from build123d import *

# Parameters (mm, degrees)
F0_R      = 3.1
F0_R_2    = 2.4
F1_DEPTH  = 87.8
F2_DEPTH  = 1
F3_DEPTH  = 8
F4_R      = 2.4
F5_DEPTH  = 25
F4_R_2    = 3.1
F6_DEPTH  = 1
F7_R      = 3.1
F7_R_2    = 2.4
F8_DEPTH  = 1
F9_R      = 2.4
F10_DEPTH = 8
F9_R_2    = 3.1
F11_DEPTH = 1
F12_DEPTH = 7
F13_R     = 2.4
F14_DEPTH = 7.9
F13_R_2   = 3.1
F15_DEPTH = 1


# Not quite as in the source:
# - a pattern or mirror of a feature is missing from the dataset's text; its kind, count and spacing are read off the source's solid


with BuildPart() as f1:
    # F0 (on Front) → F1 (new body)
    with BuildSketch(Plane.XZ):
        Polygon((4, 7.8), (0, 7.8), (-4, 7.8), (-11.9, 7.8), (-11.9, 0), (0, 0), (11.9, 0), (11.9, 7.8), align=None)
        with Locations((-7.975, 3.9)):
            Circle(F0_R, mode=Mode.SUBTRACT)
        with Locations((0, 3.9)):
            Circle(F0_R, mode=Mode.SUBTRACT)
        with Locations((7.975, 3.9)):
            Circle(F0_R, mode=Mode.SUBTRACT)
        with Locations((7.975, 3.9)):
            Circle(F0_R)
        with Locations((7.975, 3.9)):
            Circle(F0_R_2, mode=Mode.SUBTRACT)
        with Locations((0, 3.9)):
            Circle(F0_R)
        with Locations((0, 3.9)):
            Circle(F0_R_2, mode=Mode.SUBTRACT)
        with Locations((-7.975, 3.9)):
            Circle(F0_R)
        with Locations((-7.975, 3.9)):
            Circle(F0_R_2, mode=Mode.SUBTRACT)
        with Locations((-7.975, 3.9)):
            Circle(F0_R_2)
        with Locations((0, 3.9)):
            Circle(F0_R_2)
        with Locations((7.975, 3.9)):
            Circle(F0_R_2)
    extrude(amount=F1_DEPTH)

    # F0 (on Front) → F2 (cut)
    with BuildSketch(Plane.XZ):
        with Locations((7.975, 3.9)):
            Circle(F0_R)
        with Locations((7.975, 3.9)):
            Circle(F0_R_2, mode=Mode.SUBTRACT)
        with Locations((0, 3.9)):
            Circle(F0_R)
        with Locations((0, 3.9)):
            Circle(F0_R_2, mode=Mode.SUBTRACT)
        with Locations((-7.975, 3.9)):
            Circle(F0_R)
        with Locations((-7.975, 3.9)):
            Circle(F0_R_2, mode=Mode.SUBTRACT)
    extrude(amount=F2_DEPTH, mode=Mode.SUBTRACT)

    # F0 (on Front) → F3 (cut)
    with BuildSketch(Plane.XZ):
        with Locations((-7.975, 3.9)):
            Circle(F0_R_2)
        with Locations((0, 3.9)):
            Circle(F0_R_2)
        with Locations((7.975, 3.9)):
            Circle(F0_R_2)
    extrude(amount=F3_DEPTH, mode=Mode.SUBTRACT)

    # F4 (on face) → F5 (cut)
    with BuildSketch(Plane.XY.offset(7.8)):
        with Locations((-7.9, -11.9)):
            Circle(F4_R)
        with Locations((-7.9, -75.9)):
            Circle(F4_R)
        with Locations((7.9, -75.9)):
            Circle(F4_R)
        with Locations((7.9, -11.9)):
            Circle(F4_R)
    extrude(amount=-F5_DEPTH, mode=Mode.SUBTRACT)

    # F4 (on face) → F6 (cut)
    with BuildSketch(Plane.XY.offset(7.8)):
        with Locations((-7.9, -11.9)):
            Circle(F4_R_2)
        with Locations((-7.9, -11.9)):
            Circle(F4_R, mode=Mode.SUBTRACT)
        with Locations((7.9, -11.9)):
            Circle(F4_R_2)
        with Locations((7.9, -11.9)):
            Circle(F4_R, mode=Mode.SUBTRACT)
        with Locations((-7.9, -75.9)):
            Circle(F4_R_2)
        with Locations((-7.9, -75.9)):
            Circle(F4_R, mode=Mode.SUBTRACT)
        with Locations((7.9, -75.9)):
            Circle(F4_R_2)
        with Locations((7.9, -75.9)):
            Circle(F4_R, mode=Mode.SUBTRACT)
    extrude(amount=-F6_DEPTH, mode=Mode.SUBTRACT)

    # F7 (on face) → F8 (cut)
    with BuildSketch(Plane(origin=(0, 0, 0), x_dir=(1, 0, 0), z_dir=(0, 0, -1))):
        with Locations((7.9, 75.9)):
            Circle(F7_R)
        with Locations((7.9, 75.9)):
            Circle(F7_R_2, mode=Mode.SUBTRACT)
        with Locations((-7.9, 75.9)):
            Circle(F7_R)
        with Locations((-7.9, 75.9)):
            Circle(F7_R_2, mode=Mode.SUBTRACT)
        with Locations((-7.9, 11.9)):
            Circle(F7_R)
        with Locations((-7.9, 11.9)):
            Circle(F7_R_2, mode=Mode.SUBTRACT)
        with Locations((7.9, 11.9)):
            Circle(F7_R)
        with Locations((7.9, 11.9)):
            Circle(F7_R_2, mode=Mode.SUBTRACT)
    extrude(amount=-F8_DEPTH, mode=Mode.SUBTRACT)

    # F9 (on face) → F10 (cut)
    with BuildSketch(Plane.YZ.offset(11.9)):
        with Locations((-67.9, 3.9)):
            Circle(F9_R)
        with Locations((-59.9, 3.9)):
            Circle(F9_R)
        with Locations((-51.9, 3.9)):
            Circle(F9_R)
        with Locations((-43.9, 3.9)):
            Circle(F9_R)
        with Locations((-35.9, 3.9)):
            Circle(F9_R)
        with Locations((-27.9, 3.9)):
            Circle(F9_R)
        with Locations((-19.9, 3.9)):
            Circle(F9_R)
    f10 = extrude(amount=-F10_DEPTH, mode=Mode.SUBTRACT)

    # F10_copies: F10 across plane
    add(f10.mirror(Plane(origin=(0, 0, 0), x_dir=(0, 0, -1), z_dir=(-1, 0, 0))), mode=Mode.SUBTRACT)

    # F9 (on face) → F11 (cut)
    with BuildSketch(Plane.YZ.offset(11.9)):
        with Locations((-67.9, 3.9)):
            Circle(F9_R_2)
        with Locations((-67.9, 3.9)):
            Circle(F9_R, mode=Mode.SUBTRACT)
        with Locations((-59.9, 3.9)):
            Circle(F9_R_2)
        with Locations((-59.9, 3.9)):
            Circle(F9_R, mode=Mode.SUBTRACT)
        with Locations((-51.9, 3.9)):
            Circle(F9_R_2)
        with Locations((-51.9, 3.9)):
            Circle(F9_R, mode=Mode.SUBTRACT)
        with Locations((-43.9, 3.9)):
            Circle(F9_R_2)
        with Locations((-43.9, 3.9)):
            Circle(F9_R, mode=Mode.SUBTRACT)
        with Locations((-35.9, 3.9)):
            Circle(F9_R_2)
        with Locations((-35.9, 3.9)):
            Circle(F9_R, mode=Mode.SUBTRACT)
        with Locations((-27.9, 3.9)):
            Circle(F9_R_2)
        with Locations((-27.9, 3.9)):
            Circle(F9_R, mode=Mode.SUBTRACT)
        with Locations((-19.9, 3.9)):
            Circle(F9_R_2)
        with Locations((-19.9, 3.9)):
            Circle(F9_R, mode=Mode.SUBTRACT)
    f11 = extrude(amount=-F11_DEPTH, mode=Mode.SUBTRACT)

    # F11_copies: F11 across plane
    add(f11.mirror(Plane(origin=(0, 0, 0), x_dir=(0, 0, -1), z_dir=(-1, 0, 0))), mode=Mode.SUBTRACT)

    # F4 (on face) → F12 (cut)
    with BuildSketch(Plane.XY.offset(7.8)):
        Polygon((-11.1, -6.9), (-11.1, -7.9), (-3.9, -7.9), (-3.9, -15.9), (-4.9, -15.9), (-4.9, -71.9), (-3.9, -71.9), (-3.9, -79.9), (-11.1, -79.9), (-11.1, -80.9), (11.1, -80.9), (11.1, -79.9), (3.9, -79.9), (3.9, -71.9), (4.9, -71.9), (4.9, -15.9), (3.9, -15.9), (3.9, -7.9), (11.1, -7.9), (11.1, -6.9), align=None)
    extrude(amount=-F12_DEPTH, mode=Mode.SUBTRACT)

    # F13 (on face) → F14 (cut)
    with BuildSketch(Plane.XZ.offset(87.8)):
        with Locations((-8, 3.9)):
            Circle(F13_R)
        with Locations((0, 3.9)):
            Circle(F13_R)
        with Locations((8, 3.9)):
            Circle(F13_R)
    extrude(amount=-F14_DEPTH, mode=Mode.SUBTRACT)

    # F13 (on face) → F15 (cut)
    with BuildSketch(Plane.XZ.offset(87.8)):
        with Locations((-8, 3.9)):
            Circle(F13_R_2)
        with Locations((-8, 3.9)):
            Circle(F13_R, mode=Mode.SUBTRACT)
        with Locations((0, 3.9)):
            Circle(F13_R_2)
        with Locations((0, 3.9)):
            Circle(F13_R, mode=Mode.SUBTRACT)
        with Locations((8, 3.9)):
            Circle(F13_R_2)
        with Locations((8, 3.9)):
            Circle(F13_R, mode=Mode.SUBTRACT)
    extrude(amount=-F15_DEPTH, mode=Mode.SUBTRACT)


solid = f1.part
Can you work these out from the model? Positions are in its coordinate system, mm. A direction names the side the tool comes from. Give positions to 0.01 mm unless a question says otherwise; leave off trailing zeros. Loops run counter-clockwise (first coordinate to the right, second up) from the corner with the lowest first, then second, coordinate; pieces in that order, holes last. Notation, with made-up numbers: (62, -38) -> (95, -38) arc R38 cw to (95, 1) -> close; hole circle Ø2 at (21, 24). An arc over 180 degrees is marked (long way). Write item = value, one per line.
1) Suppose I cut it at A-A on y = -11.9. Give the number of separate pieces and of enclosed holes in the cut face, then the cut area to 3 significant figures.
Check result:
separate_pieces = 3
enclosed_holes = 0
area = 50.6 mm2
2) For faces 5 (the flat face through (-10.9, -66, 2)), 6 (the cylindrical face through (7.496, -78.974, 0.493)), 7 (the flat face through (-6, -14, 6.8)), 8 (the cylindrical face through (4.9, -87.3, 4)), 9 (the flat face through (8, -8, 4)), which set-ups out of +Z, -Z, +X, -X, +Y, -Y let a thin tool reach every point of the face, with its end or its side?
Check result:
face_5 = -X
face_6 = -Z
face_7 = +Z
face_8 = -Y
face_9 = +Y
3) I need wall thicknesses on L1, parallel to X at y = -11.9, z = 5.1; L2, parallel to X at y = -47, z = 6.75; L3, parallel to X at y = -7.5, z = 5. Which ranges of each line are inside material? Lowest first, please. Write a range as from..to.
Check result:
L1 = -11.9..-10.3, -5.5..-3.9, 3.9..5.5, 10.3..11.9
L2 = -11.9..-4.9, 4.9..11.9
L3 = -11.9..-11.1, 11.1..11.9
4) Thinking about a two-plate mould opening in Z: for faces 1 (the cylindrical face through (11.41, -18.23, 6.51)), 2 (the flat face through (-4.9, -44, 7)), 3 (the flat face through (0, -43, 0)), 4 (the cylindrical face through (11.4, -47, 4)), which applies, released by +Z, released by -Z, zero draft, split by the parting line, or undercut?
Check result:
face_1 = undercut
face_2 = zero draft
face_3 = released by -Z
face_4 = undercut
5) Will these pins go through, and if not, where does the flat tip stop? pin 1 (6 mm diameter, centred on x = -7.9, y = -11.9, fed in from +Z); pin 2 (1.4 mm diameter, centred on x = -7, z = 3.5, fed in from +Y); pin 3 (6.5 mm diameter, centred on x = -1.5, y = -37, fed in from +Z).
Check result:
pin_1 = 6.8
pin_2 = -8
pin_3 = 0.8
6) Suppose I cut it at B-B on x = 0. Write out the boundary of the cut face in (y, z).
Check result:
outline = (-87.8, 0) -> (0, 0) -> (0, 0.8) -> (-1, 0.8) -> (-1, 1.5) -> (-6.9, 1.5) -> (-6.9, 0.8) -> (-80.9, 0.8) -> (-80.9, 1.5) -> (-86.8, 1.5) -> (-86.8, 0.8) -> (-87.8, 0.8) -> close; (-87.8, 7) -> (-86.8, 7) -> (-86.8, 6.3) -> (-80.9, 6.3) -> (-80.9, 7.8) -> (-87.8, 7.8) -> close; (-6.9, 6.3) -> (-1, 6.3) -> (-1, 7) -> (0, 7) -> (0, 7.8) -> (-6.9, 7.8) -> close
7) Suppose I cut it at C-C on y = -59.9. Write out the boundary of the cut face in (x, z), then the cut area to 3 significant figures.
Check result:
outline = (-11.9, 0) -> (11.9, 0) -> (11.9, 0.8) -> (10.9, 0.8) -> (10.9, 1.5) -> (4.9, 1.5) -> (4.9, 0.8) -> (-4.9, 0.8) -> (-4.9, 1.5) -> (-10.9, 1.5) -> (-10.9, 0.8) -> (-11.9, 0.8) -> close; (-11.9, 7) -> (-10.9, 7) -> (-10.9, 6.3) -> (-4.9, 6.3) -> (-4.9, 7.8) -> (-11.9, 7.8) -> close; (4.9, 6.3) -> (10.9, 6.3) -> (10.9, 7) -> (11.9, 7) -> (11.9, 7.8) -> (4.9, 7.8) -> close
area = 47.0 mm2
